from build123d import *
from build123d.topology import SkipClean

# Parameters (mm, degrees)
SKETCH_1_R               = 19.5
EXTRUDE_1_DEPTH          = 22
CUT_EXTRUDE_1_DEPTH      = 61.170590823
CUT_EXTRUDE_1_DEPTH_BACK = 61.170590823
SKETCH_2_R               = 10
CUT_EXTRUDE_START        = -2.5
CUT_EXTRUDE_2_DEPTH      = 2.5
EXTRUDE_START            = -22
EXTRUDE_2_DEPTH          = 22
CUT_EXTRUDE_4_DEPTH      = 61.170590823
CUT_EXTRUDE_4_DEPTH_BACK = 61.170590823
SKETCH_5_R               = 6.5
CUT_EXTRUDE_5_DEPTH      = 2.5
FILLET_1_R               = 1
CUT_EXTRUDE_6_DEPTH      = 2.5


with BuildPart() as part:
    # 草图1 → 凸台-拉伸1 (new body)
    with BuildSketch(Plane(origin=(0, 0, 0), x_dir=(1, 0, 0), z_dir=(0, 1, 0))):
        Circle(SKETCH_1_R)
        with Locations((0, -33)):
            Circle(SKETCH_1_R)
    extrude(amount=EXTRUDE_1_DEPTH)

    # 草图2 → 切除-拉伸1 (cut, two sides: drawn at the far end of the back side and taken through both)
    with BuildSketch(Plane(origin=(0, 22, 0), x_dir=(1, 0, 0), z_dir=(0, 1, 0)).offset(-CUT_EXTRUDE_1_DEPTH_BACK)):
        with Locations(Location((0, 0, 0), (0, 0, 270))):
            Circle(SKETCH_2_R)
        with Locations(Location((0, -33, 0), (0, 0, 270))):
            Circle(SKETCH_2_R)
    extrude(amount=CUT_EXTRUDE_1_DEPTH + CUT_EXTRUDE_1_DEPTH_BACK, mode=Mode.SUBTRACT)

    # 草图3 → 切除-拉伸2 (cut)
    with BuildSketch(Plane(origin=(0, 22, 0), x_dir=(1, 0, 0), z_dir=(0, 1, 0)).offset(CUT_EXTRUDE_START)):
        with BuildLine():
            Line((-16.887495374, 9.75), (-12.369316877, 7.141428429))
            ThreePointArc((-12.369316877, 7.141428429), (-10.683653707, 6.844745078), (-9.202193277, 7.701924362))
            ThreePointArc((-9.202193277, 7.701924362), (10.872513333, 5.078233337), (0, -12))
            ThreePointArc((0, -12), (-4.5, -16.5), (0, -21))
            ThreePointArc((0, -21), (10.872513333, -38.078233337), (-9.202193277, -40.701924362))
            ThreePointArc((-9.202193277, -40.701924362), (-10.683653707, -39.844745078), (-12.369316877, -40.141428429))
            Line((-12.369316877, -40.141428429), (-16.887495374, -42.75))
            ThreePointArc((-16.887495374, -42.75), (-15.186446596, -45.232000645), (-13.123802868, -47.422752799))
            Line((-13.123802868, -47.422752799), (-11.421452311, -45.551909301))
            ThreePointArc((-11.421452311, -45.551909301), (-10.758297788, -45.227853244), (-10.053481376, -45.446988078))
            ThreePointArc((-10.053481376, -45.446988078), (15.085619133, -38.331425267), (0, -17))
            ThreePointArc((0, -17), (-0.5, -16.5), (0, -16))
            ThreePointArc((0, -16), (15.085619133, 5.331425267), (-10.053481376, 12.446988078))
            ThreePointArc((-10.053481376, 12.446988078), (-10.758297788, 12.227853244), (-11.421452311, 12.551909301))
            Line((-11.421452311, 12.551909301), (-13.123802868, 14.422752799))
            ThreePointArc((-13.123802868, 14.422752799), (-15.186446596, 12.232000645), (-16.887495374, 9.75))
        make_face()
    extrude(amount=CUT_EXTRUDE_2_DEPTH, mode=Mode.SUBTRACT)

    # 草图4 → 凸台-拉伸2 (add)
    with BuildSketch(Plane(origin=(0, 22, 0), x_dir=(1, 0, 0), z_dir=(0, 1, 0)).offset(EXTRUDE_START)):
        with BuildLine():
            ThreePointArc((11.012786163, -16.907500476), (11, -16.5), (11.012786163, -16.092499524))
            ThreePointArc((11.012786163, -16.092499524), (10.704484781, -16.299202605), (10.392304845, -16.5))
            ThreePointArc((10.392304845, -16.5), (10.704484781, -16.700797395), (11.012786163, -16.907500476))
        make_face()
        with BuildLine():
            ThreePointArc((-11.012786163, -16.092499524), (-11.003197327, -16.296149488), (-11, -16.5))
            ThreePointArc((-11, -16.5), (-11.003197327, -16.703850512), (-11.012786163, -16.907500476))
            ThreePointArc((-11.012786163, -16.907500476), (-10.704484781, -16.700797395), (-10.392304845, -16.5))
            ThreePointArc((-10.392304845, -16.5), (-10.704484781, -16.299202605), (-11.012786163, -16.092499524))
        make_face()
    extrude(amount=EXTRUDE_2_DEPTH)

    # 草图5 → 切除-拉伸4 (cut, two sides: drawn at the far end of the back side and taken through both)
    with SkipClean():  # the faces are left unmerged after this step: merging them gives an invalid solid
        with BuildSketch(Plane(origin=(0, 22, 0), x_dir=(1, 0, 0), z_dir=(0, 1, 0)).offset(-CUT_EXTRUDE_4_DEPTH_BACK)):
            with Locations((17.5, -16.5)):
                Circle(SKETCH_5_R)
            with Locations((-17.5, -16.5)):
                Circle(SKETCH_5_R)
        extrude(amount=CUT_EXTRUDE_4_DEPTH + CUT_EXTRUDE_4_DEPTH_BACK, mode=Mode.SUBTRACT)

    # 草图6 → 切除-拉伸5 (cut)
    with SkipClean():  # the faces are left unmerged after this step: merging them gives an invalid solid
        with BuildSketch(Plane.XZ.offset(CUT_EXTRUDE_START)):
            with BuildLine():
                Line((-12.376524617, 12.5), (-2, 12.5))
                Line((-2, 12.5), (-2, 20.5))
                Line((-2, 20.5), (-12.376524617, 20.5))
                ThreePointArc((-12.376524617, 20.5), (-11, 16.5), (-12.376524617, 12.5))
            make_face()
            with BuildLine():
                Line((2, 20.5), (2, 12.5))
                Line((2, 12.5), (12.376524617, 12.5))
                ThreePointArc((12.376524617, 12.5), (11, 16.5), (12.376524617, 20.5))
                Line((12.376524617, 20.5), (2, 20.5))
            make_face()
        extrude(amount=CUT_EXTRUDE_5_DEPTH, mode=Mode.SUBTRACT)

    # 圆角1
    fillet_1_edges = [part.edges().sort_by_distance(p)[0] for p in [
        (-2, 1.25, 20.5),
        (-2, 1.25, 12.5),
        (2, 1.25, 20.5),
        (2, 1.25, 12.5),
    ]]
    fillet(fillet_1_edges, radius=FILLET_1_R)

    # 草图7 → 切除-拉伸6 (cut)
    with SkipClean():  # the faces are left unmerged after this step: merging them gives an invalid solid
        with BuildSketch(Plane(origin=(0, 22, 0), x_dir=(1, 0, 0), z_dir=(0, 1, 0))):
            Polygon((-94.212388388, -97.040815513), (-15.085786438, -17.914213562), (1.414213562, -1.414213562), (-1.414213562, 1.414213562), (-17.914213562, -15.085786438), (-19.328427125, -16.5), (-15.503778834, -20.324648291), (-1.414213562, -34.414213562), (1.414213562, -31.585786438), (-13.671572875, -16.5), (-92.798174826, 62.62660195), (-316.593223793, 64.608809708), (-318.007437355, -95.058607756), align=None)
        extrude(amount=-CUT_EXTRUDE_6_DEPTH, mode=Mode.SUBTRACT)


solid = part.part
The model under review builds one solid part; all positions refer to its coordinate system, in mm. A direction names the side the tool comes from. Round coordinates to 2 decimals unless told otherwise and drop trailing zeros. Loops run counter-clockwise (first coordinate to the right, second up) from the corner with the lowest first, then second, coordinate; pieces in that order, holes last. Notation, with made-up numbers: (11.25, 84.5) -> (26.25, 84.5) arc R21 ccw to (26.25, 99.5) -> close; hole circle Ø5 at (86.25, 87). An arc over 180 degrees is marked (long way). Write item = value, one per line. Start each with the question number.
Item 1: To check wall thickness, follow L1, parallel to X at y = 21.05, z = 33; L2, parallel to Z at x = 0, y = 14.75; L3, parallel to Z at x = -9, y = 6.5. State the ranges of each line that lie inside material, in increasing order.
Item 2: Take a section at B-B on y = 18. Give the boundary of the cut face in (x, z).
Item 3: Insertion check: pin 1 (3 mm diameter, centred on y = 1.5, z = 16, fed in from +X); pin 2 (3 mm diameter, centred on x = 9, y = 0.5, fed in from +Z); pin 3 (3 mm diameter, centred on x = 4.5, y = 16, fed in from +Z). Each pin has a flat end and moves straight along its axis. Give the tip position at first contact, or say it passes through.
Item 4: Take a section at A-A on z = 0. Give the boundary of the cut face in (x, y).
Item 5: Take a section at C-C on x = -7. Give the boundary of the cut face in (y, z), plus the area to 3 significant figures.
Item 6: For faces 3 (the cylindrical face through (-10.71, 20.73, -6.84)), 4 (the flat face through (-8, 1, 20.5)), 5 (the flat face through (9, 22, 19)), 6 (the flat face through (-12.285, 20.732, 46.5)), list the 3-axis set-ups (+Z, -Z, +X, -X, +Y, -Y) from which the entire face can be reached by the end or side of a thin tool; tool diameter is ignored.
Item 7: Mouldability with a two-part tool opening along Z and no side actions: class faces 1 (the flat face through (-7, 22, 16)), 2 (the flat face through (-11.17, 20.77, 24.66)) as released by +Z, released by -Z, zero draft, split by the parting line, or undercut.
Item 8: Take a section at D-D on x = -15. Give the boundary of the cut face in (y, z).
Result:
q1.L1 = -19.5 to -10, 10 to 12, 16 to 19.5
q1.L2 = -19.5 to -10, 10 to 23, 43 to 52.5
q1.L3 = -17.3 to -4.36, 4.36 to 28.64, 37.36 to 50.3
q2.outline = (-16.71, 10.05) arc R19.5 ccw (long way) to (16.71, 10.05) arc R6.5 cw to (16.71, 22.95) arc R19.5 ccw (long way) to (-16.71, 22.95) arc R6.5 cw to start; hole circle Ø20 at (0, 0); hole circle Ø20 at (0, 33)
q3.pin_1 = 11.2
q3.pin_2 = 51
q3.pin_3 = 52.27
q4.outline = (-19.5, 0) -> (-10, 0) -> (-10, 22) -> (-19.5, 22) -> close; (10, 0) -> (19.5, 0) -> (19.5, 22) -> (16, 22) -> (16, 19.5) -> (12, 19.5) -> (12, 22) -> (10, 22) -> close
q5.outline = (0, -18.2) -> (22, -18.2) -> (22, -14.39) -> (19.5, -14.39) -> (19.5, -9.75) -> (22, -9.75) -> (22, -7.14) -> (0, -7.14) -> close; (0, 7.14) -> (19.5, 7.14) -> (19.5, 9.83) -> (22, 9.83) -> (22, 23.17) -> (19.5, 23.17) -> (19.5, 25.86) -> (0, 25.86) -> (0, 20.5) -> (2.5, 20.5) -> (2.5, 12.5) -> (0, 12.5) -> close; (0, 40.14) -> (22, 40.14) -> (22, 42.75) -> (19.5, 42.75) -> (19.5, 47.39) -> (22, 47.39) -> (22, 51.2) -> (0, 51.2) -> close
q5.area = 842 mm²
q6.face_3 = +Y
q6.face_4 = -X, -Y
q6.face_5 = +Z, -Z, +X, -X, +Y
q6.face_6 = -X, +Y
q7.face_1 = zero draft
q7.face_2 = undercut
q8.outline = (0, -12.46) -> (19.5, -12.46) -> (19.5, -8.66) -> (22, -8.66) -> (22, 10.5) -> (0, 10.5) -> close; (0, 22.5) -> (22, 22.5) -> (22, 41.66) -> (19.5, 41.66) -> (19.5, 45.46) -> (0, 45.46) -> close
